CAD build for the part. Positions are in the model's coordinates, mm. Give positions to 0.01 mm unless a question says otherwise; leave off trailing zeros. Write each loop counter-clockwise with the first axis right and the second up, starting at its lowest first coordinate (ties: lowest second). Pieces come first, ordered by that corner, then holes. Notation, with made-up numbers: (76.5, -14) - (125.5, -14) arc R24 cw to (125.5, -1) - close; hole circle Ø4 at (7, 54.5). An arc over 180 degrees is marked (long way). Put each result on its own line as item: value. Start each with the question number.
1. Cut at A-A on z = 257.5. List the corners of the cut face in (x, y), and give its area (3 significant figures).
2. Drop flat-ended pins along their axis: pin 1 (0.9 mm diameter, centred on x = 5.5, z = 190.5, fed in from +Y); pin 2 (0.9 mm diameter, centred on y = 5, z = 145.5, fed in from +X). Give the stop position or say it passes through.
3. Wall check: line 1 (X direction, y = 10, z = 9.25); line 2 (Y direction, x = 14, z = 6.75); line 3 (Y direction, x = 5.25, z = 218). Give the ranges that are in metal, low to high.
from build123d import *

# Parameters (mm, degrees)
SZKIC1_W                       = 25
SZKIC1_H                       = 25
DODANIE_WYCI_GNI_CIE1_DEPTH    = 500
SZKIC2_W                       = 3
SZKIC2_H                       = 464
WYTNIJ_WYCI_GNI_CIE1_DEPTH     = 3
SZKIC3_W                       = 464
SZKIC3_H                       = 3
WYTNIJ_WYCI_GNI_CIE2_DEPTH     = 3
OTWORY_USTALAJ_CE_3_0MM1_D     = 3
OTWORY_USTALAJ_CE_3_0MM1_DEPTH = 16
OTWORY_USTALAJ_CE_3_0MM1_TIP   = 0.901290929


with BuildPart() as part:
    # Szkic1 → Dodanie-wyciągnięcie1 (new body)
    with BuildSketch(Plane.XY):
        with Locations((12.5, 12.5)):
            Rectangle(SZKIC1_W, SZKIC1_H)
    extrude(amount=DODANIE_WYCI_GNI_CIE1_DEPTH)

    # Szkic2 → Wytnij-wyciągnięcie1 (cut)
    with BuildSketch(Plane(origin=(0, 25, 0), x_dir=(1, 0, 0), z_dir=(0, 1, 0))):
        with Locations((5, -250)):
            Rectangle(SZKIC2_W, SZKIC2_H)
    extrude(amount=-WYTNIJ_WYCI_GNI_CIE1_DEPTH, mode=Mode.SUBTRACT)

    # Szkic3 → Wytnij-wyciągnięcie2 (cut)
    with BuildSketch(Plane(origin=(25, 0, 0), x_dir=(0, 0, -1), z_dir=(1, 0, 0))):
        with Locations((-250, 5)):
            Rectangle(SZKIC3_W, SZKIC3_H)
    extrude(amount=-WYTNIJ_WYCI_GNI_CIE2_DEPTH, mode=Mode.SUBTRACT)

    # Otwory ustalające Ø3.0mm1
    with Locations(Plane(origin=(0, 0, 0), x_dir=(-1, 0, 0), z_dir=(0, 0, -1))):
        with Locations((-14, 10)):
            Hole(OTWORY_USTALAJ_CE_3_0MM1_D / 2, depth=OTWORY_USTALAJ_CE_3_0MM1_DEPTH)
            with Locations((0, 0, -(OTWORY_USTALAJ_CE_3_0MM1_DEPTH + OTWORY_USTALAJ_CE_3_0MM1_TIP / 2))):  # 118° drill point
                Cone(0, OTWORY_USTALAJ_CE_3_0MM1_D / 2, OTWORY_USTALAJ_CE_3_0MM1_TIP, mode=Mode.SUBTRACT)


solid = part.part
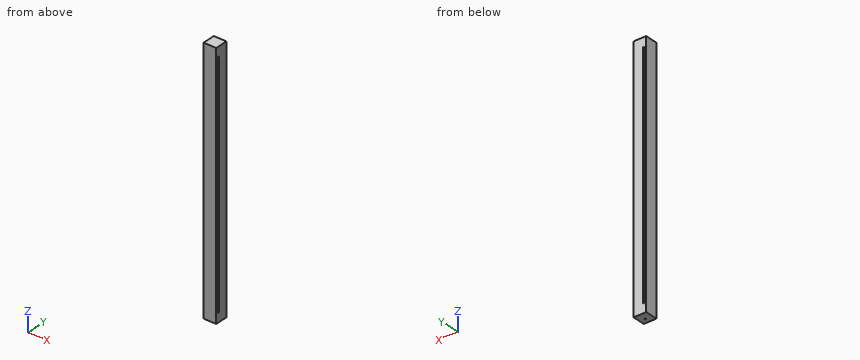
Report:
1. outline: (0, 0) - (25, 0) - (25, 3.5) - (22, 3.5) - (22, 6.5) - (25, 6.5) - (25, 25) - (6.5, 25) - (6.5, 22) - (3.5, 22) - (3.5, 25) - (0, 25) - close
1. area: 607 mm²
2. pin 1: stops at y = 22
2. pin 2: stops at x = 22
3. line 1: x = 0 to 12.5, 15.5 to 25
3. line 2: y = 0 to 8.5, 11.5 to 25
3. line 3: y = 0 to 22
